Read the model definition and answer for the solid it produces. Units are mm, in the model's axes. Face numbers are marked on the shaded views. A direction names the side the tool comes from. Round coordinates to 2 decimals unless told otherwise and drop trailing zeros. Loops run counter-clockwise (first coordinate to the right, second up) from the corner with the lowest first, then second, coordinate; pieces in that order, holes last. Notation, with made-up numbers: (-1.75, -35.75) -> (42.25, -35.75) arc R37 cw to (42.25, 3.25) -> close; hole circle Ø10 at (-14, 68). An arc over 180 degrees is marked (long way). Put each result on its own line as item: value.
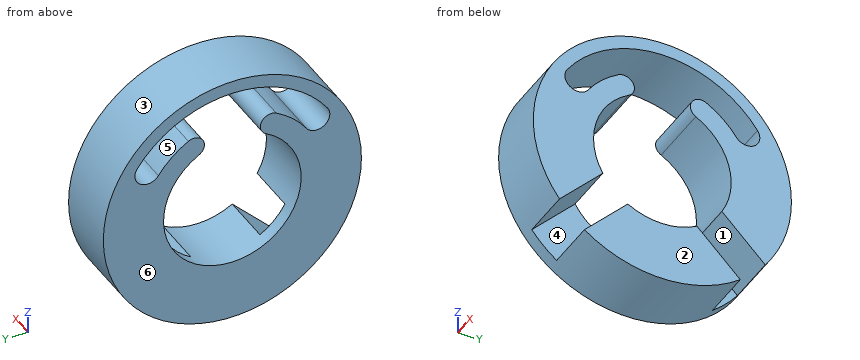
from build123d import *

# Parameters (mm, degrees)
SKETCH087_R             = 8
SKETCH087_R_2           = 4
PAD045_DEPTH            = 7.5
SKETCH088_R             = 6
SKETCH088_R_2           = 4
PAD046_DEPTH            = 7
SKETCH089_R             = 8
SKETCH089_R_2           = 4
PAD047_DEPTH            = 1.5
SKETCH090_R             = 2
PAD048_DEPTH            = 9
BODY031_ROLL_ANGLE      = 45
BODY031_PLACEMENT_ANGLE = 180
SKETCH091_R             = 15
PAD049_DEPTH            = 3.75
POCKET029_DEPTH         = 6
POLARPATTERN021_COUNT   = 2
POLARPATTERN021_ANGLE   = 90


with BuildPart() as polea8d:
    # Sketch087 → Pad045 (new body)
    with BuildSketch(Plane.YZ):
        Circle(SKETCH087_R)
        Circle(SKETCH087_R_2, mode=Mode.SUBTRACT)
    extrude(amount=PAD045_DEPTH)

    # Sketch088 (on Face3 of Pad045) → Pad046 (join)
    with BuildSketch(Plane(origin=(0, 0, 0), x_dir=(0, 1, 0), z_dir=(-1, 0, 0))):
        Circle(SKETCH088_R)
        Circle(SKETCH088_R_2, mode=Mode.SUBTRACT)
    extrude(amount=PAD046_DEPTH)

    # Sketch089 (on Face6 of Pad046) → Pad047 (join)
    with BuildSketch(Plane(origin=(-7, 0, 0), x_dir=(0, 1, 0), z_dir=(-1, 0, 0))):
        Circle(SKETCH089_R)
        Circle(SKETCH089_R_2, mode=Mode.SUBTRACT)
    extrude(amount=PAD047_DEPTH)

    # Sketch090 → Pad048 (join)
    with BuildSketch(Plane.XZ):
        with Locations((4, 0)):
            Circle(SKETCH090_R)
    extrude(amount=PAD048_DEPTH)


with BuildPart() as polea8d_1:
    # Body031 roll: moved
    add(polea8d.part.rotate(Axis((0, 0, 0), (1, 0, 0)), BODY031_ROLL_ANGLE))


with BuildPart() as polea8d_2:
    # Body031 placement: moved
    add(polea8d_1.part.moved(Location((22.5, 0, 0))).rotate(Axis((22.5, 0, 0), (0, 0, 1)), BODY031_PLACEMENT_ANGLE))


with BuildPart() as body034:
    # Sketch091 → Pad049 (new body, symmetric)
    with BuildSketch(Plane.YZ):
        Circle(SKETCH091_R)
        with BuildLine():
            ThreePointArc((-3.891892, 6.989505), (0, -8), (3.891892, 6.989505))
            ThreePointArc((5.108116, 9.17372), (3.407892, 8.689727), (3.891892, 6.989505))
            ThreePointArc((8.601093, 6.022558), (7.033353, 7.796277), (5.108116, 9.17372))
            ThreePointArc((8.601093, 6.022558), (10.690187, 5.654187), (11.058552, 7.743282))
            ThreePointArc((11.058552, 7.743282), (0, 13.5), (-11.058553, 7.743282))
            ThreePointArc((-11.058553, 7.743282), (-10.690189, 5.654189), (-8.601096, 6.022553))
            ThreePointArc((-5.108108, 9.173725), (-7.033352, 7.796278), (-8.601096, 6.022553))
            ThreePointArc((-3.891892, 6.989505), (-3.40789, 8.689723), (-5.108108, 9.173725))
        make_face(mode=Mode.SUBTRACT)
    extrude(amount=PAD049_DEPTH, both=True)


with BuildPart() as body034_1:
    # Body032 placement: moved
    add(body034.part.moved(Location((18.5, 0, 0))))

    # Cut005: cut polea8d
    add(polea8d_2.part, mode=Mode.SUBTRACT)

    # Sketch092 (on Face3 of BaseFeature005) → Pocket029 (cut)
    with BuildSketch(Plane.YZ.offset(22.25)):
        Polygon((4.018406, -6.917544), (9.86414, -12.763277), (12.763277, -9.86414), (6.917544, -4.018406), align=None)
    pocket029 = extrude(amount=-POCKET029_DEPTH, mode=Mode.SUBTRACT)

    # PolarPattern021: Pocket029 ×2 about axis
    polarpattern021_axis = Axis((22.25, 0, 0), (-1, 0, 0))
    for i in range(1, POLARPATTERN021_COUNT):
        add(pocket029.rotate(polarpattern021_axis, i * POLARPATTERN021_ANGLE / (POLARPATTERN021_COUNT - 1)), mode=Mode.SUBTRACT)


solid = body034_1.part
Item 1: The part is cut by section D-D (y = -4.5). Determine the outline of the cut face in (x, z), then the cut area to 3 significant figures.
Derived:
outline: (14.75, -14.31) -> (22.25, -14.31) -> (22.25, -7.4) -> (16.25, -7.4) -> (16.25, -6.61) -> (14.75, -6.61) -> close; (14.75, 6.61) -> (22.25, 6.61) -> (22.25, 9.33) -> (14.75, 9.33) -> close; (14.75, 12.73) -> (22.25, 12.73) -> (22.25, 14.31) -> (14.75, 14.31) -> close
area: 85.2 mm^2
Item 2: The part is cut by section B-B (z = 0). Determine the outline of the cut face in (x, y), then the cut area to 3 significant figures.
Derived:
outline: (14.75, -15) -> (22.25, -15) -> (22.25, -8) -> (14.75, -8) -> close; (14.75, 8) -> (22.25, 8) -> (22.25, 15) -> (14.75, 15) -> close
area: 105 mm^2
Item 3: Find the intervals of material crossed by line 1 along Y through (x, z) = (20.5, 0); line 2 along Z through (x, y) = (19.25, 6.5); line 3 along Z through (x, y) = (20.75, 3.75), in increasing order.
Derived:
line 1: y = -15 to -8, 8 to 15
line 2: z = -13.52 to -9.4, 4.66 to 8.25, 11.83 to 13.52
line 3: z = -14.52 to -7.07, 7.08 to 9.08, 12.97 to 14.52
Item 4: The part is cut by section A-A (y = 0). Determine the outline of the cut face in (x, z).
Derived:
outline: (14.75, -15) -> (22.25, -15) -> (22.25, -8) -> (14.75, -8) -> close; (14.75, 13.5) -> (22.25, 13.5) -> (22.25, 15) -> (14.75, 15) -> close
Item 5: For a pull along Y with two mould halves and no side action, classify the marked faces 1, 2 and 3 as pulls with the +Y half, pulls with the -Y half, needs draft (parallel to the pull), parting line crosses it, or undercut.
Derived:
face 1: undercut
face 2: needs draft
face 3: parting line crosses it
Item 6: Flat-ended cylindrical pins translate along their axes: pin 1 Ø3 at (x, z) = (19, -4) entering from -Y; pin 2 Ø2 at (x, y) = (17.5, 11) entering from -Z. Find the tip coordinate at first contact, or state that the pin passes through.
Derived:
pin 1: stops at y = -14.79
pin 2: stops at z = -9.06
Item 7: The part is cut by section C-C (x = 21.25). Determine the outline of the cut face in (y, z).
Derived:
outline: (-11.96, -9.06) -> (-6.92, -4.02) arc R8 cw to (-3.89, 6.99) arc R1.25 ccw to (-5.11, 9.17) arc R10.5 ccw to (-8.6, 6.02) arc R1.5 cw to (-11.06, 7.74) arc R13.5 cw to (11.06, 7.74) arc R1.5 cw to (8.6, 6.02) arc R10.5 ccw to (5.11, 9.17) arc R1.25 ccw to (3.89, 6.99) arc R8 cw to (6.92, -4.02) -> (11.96, -9.06) arc R15 ccw (long way) to start; (-9.06, -11.96) arc R15 ccw to (9.06, -11.96) -> (4.02, -6.92) arc R8 cw to (-4.02, -6.92) -> close
Item 8: Which of the six approach directions +Z, -Z, +X, -X, +Y, -Y give full straight-line access (tool end or side, diameter ignored) to the marked faces 4, 5 and 6?
Derived:
face 4: +X
face 5: +X, -X
face 6: +Z, -Z, -X, +Y, -Y
